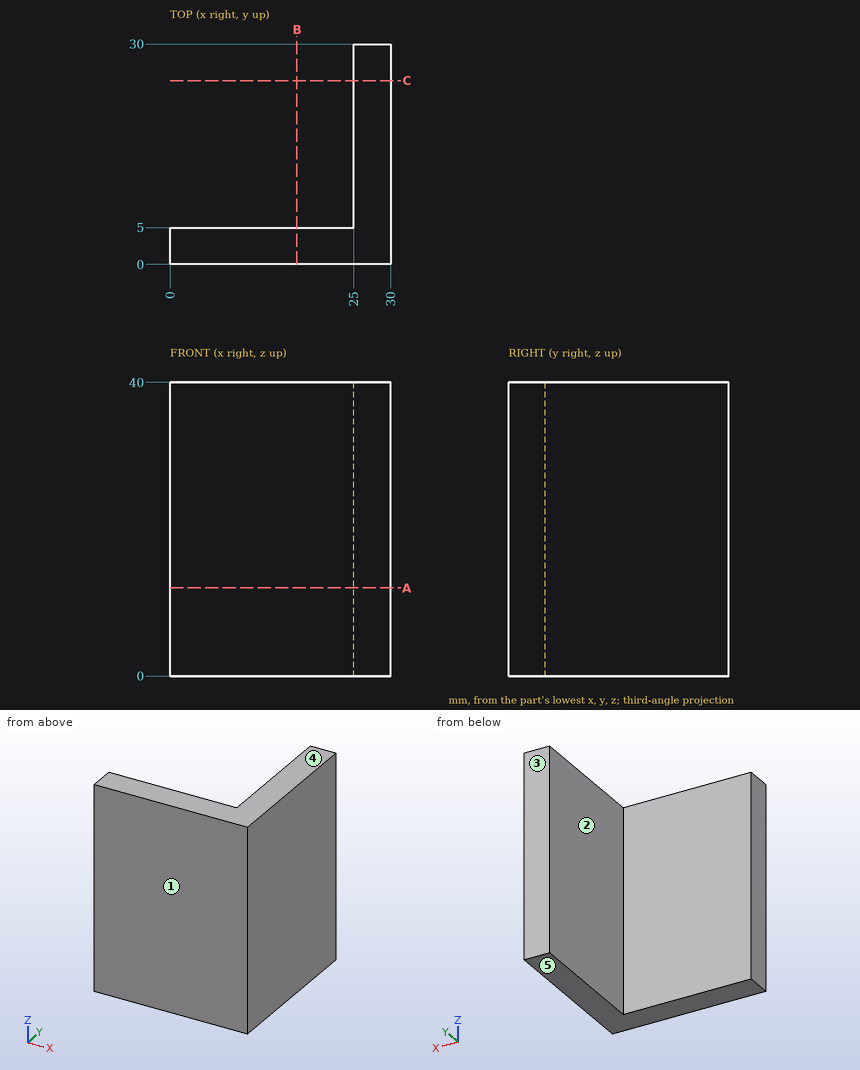
Job drawing, mm, ordinate dimensions from the low corner. One solid piece. A direction names the side the tool comes from. Give positions to 0.01 mm unless a question says otherwise; leave off trailing zeros. Order: outer loops, then holes, each group sorted by start corner. A loop starts at its lowest first (then second) coordinate and runs counter-clockwise, first axis right, second up. Notation, with made-up numbers: (39, 29) -> (68, 29) arc R30 ccw to (68, 55) -> close; hole circle Ø4 at (-29.5, -40). An arc over 180 degrees is marked (long way). Return JSON: item names as keys, results as strings.
Q1. Drill centre lines: line 1 (Y direction, x = 12, z = 8); line 2 (X direction, y = 18, z = 2). Where is each one in solid material? Low to high.
Working result:
{"line 1": "0 to 5", "line 2": "25 to 30"}
Q2. Saw through at C-C (y = 25). Write the cut outline in (x, z), then the cut area to 3 significant figures.
Working result:
{"outline": "(25, 0) -> (30, 0) -> (30, 40) -> (25, 40) -> close", "area": "200 mm²"}
Q3. Saw through at B-B (x = 17.25). Write the cut outline in (y, z), then the cut area to 3 significant figures.
Working result:
{"outline": "(0, 0) -> (5, 0) -> (5, 40) -> (0, 40) -> close", "area": "200 mm²"}
Q4. Mould opens along Z. For the marked faces 3, 4 and 5 say: pulls with the +Z half, pulls with the -Z half, needs draft (parallel to the pull), parting line crosses it, or undercut.
Working result:
{"face 3": "needs draft", "face 4": "pulls with the +Z half", "face 5": "pulls with the -Z half"}
Q5. Which spindle directions (+Z, -Z, +X, -X, +Y, -Y) get a long thin tool onto all of the face, cutting with end or side? Do the marked faces 1 and 2. Say none if no direction does.
Working result:
{"face 1": "+Z, -Z, +X, -X, -Y", "face 2": "+Z, -Z, -X, +Y"}
Q6. Flat gauge pins, fed straight in: pin 1 (4 mm diameter, centred on x = 20, z = 7, fed in from +Y); pin 2 (6 mm diameter, centred on x = 4.5, z = 7, fed in from -Y). Where does each tip first touch, or does it go through?
Working result:
{"pin 1": "y = 5", "pin 2": "y = 0"}
Q7. Saw through at A-A (z = 12). Write the cut outline in (x, y).
Working result:
{"outline": "(0, 0) -> (30, 0) -> (30, 30) -> (25, 30) -> (25, 5) -> (0, 5) -> close"}
